Could you check a few things on this model? Use its own coordinates, in mm. Face numbers are marked on the shaded views. Round coordinates to 2 decimals unless told otherwise and drop trailing zeros. Write each loop counter-clockwise with the first axis right and the second up, starting at its lowest first coordinate (ties: lowest second). Pieces come first, ordered by that corner, then holes.
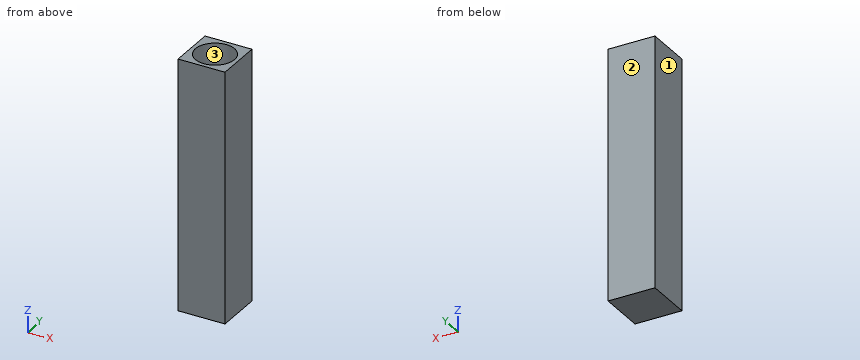
```python
from build123d import *

# Parameters (mm, degrees)
SKETCH1_W           = 76.2
SKETCH1_H           = 76.2
SKETCH1_R           = 31.75
BOSS_EXTRUDE1_DEPTH = 406.4
CUT_EXTRUDE1_START  = 406.4
SKETCH1_3_R         = 31.75
CUT_EXTRUDE1_DEPTH  = 304.8


with BuildPart() as part:
    # Sketch1 → Boss-Extrude1 (new body)
    with BuildSketch(Plane.XY):
        Rectangle(SKETCH1_W, SKETCH1_H)
        Circle(SKETCH1_R, mode=Mode.SUBTRACT)
        Circle(SKETCH1_R)
    extrude(amount=BOSS_EXTRUDE1_DEPTH)

    # Sketch1<3> → Cut-Extrude1 (cut)
    with BuildSketch(Plane.XY.offset(CUT_EXTRUDE1_START)):
        Circle(SKETCH1_3_R)
    extrude(amount=-CUT_EXTRUDE1_DEPTH, mode=Mode.SUBTRACT)


solid = part.part
```
Q1. Imagine slicing it at A-A, the plane y = -5.5. Write out the boundary of the cut face in (x, z), then the cut area to 3 significant figures.
Q2. Imagine slicing it at B-B, the plane x = 0. Write out the boundary of the cut face in (y, z), then the cut area to 3 significant figures.
Q3. If I drill on L1, parallel to Y at x = 0.5, z = 133.5; L2, parallel to Z at x = 24, y = 15.5; L3, parallel to X at y = -25, z = 248, over which ranges is the centre line in solid material (lowest first)?
Q4. We'd pull the mould along X, two halves only. Please class the marked faces 1, 2 and 3: pulls with the +X half, pulls with the -X half, needs draft (parallel to the pull), parting line crosses it, or undercut.
Q5. I'm going to push flat-ended pins straight in: pin 1 Ø12 at (x, y) = (13.5, -29) entering from -Z; pin 2 Ø1.5 at (x, y) = (-18.5, -3) entering from +Z. Where does each tip first touch, or does it pass through?
Results found:
1. outline: (-38.1, 0) - (38.1, 0) - (38.1, 406.4) - (31.27, 406.4) - (31.27, 101.6) - (-31.27, 101.6) - (-31.27, 406.4) - (-38.1, 406.4) - close
1. area: 11,900 mm2
2. outline: (-38.1, 0) - (38.1, 0) - (38.1, 406.4) - (31.75, 406.4) - (31.75, 101.6) - (-31.75, 101.6) - (-31.75, 406.4) - (-38.1, 406.4) - close
2. area: 11,600 mm2
3. L1: y = -38.1 to -31.75, 31.75 to 38.1
3. L2: z = 0 to 101.6
3. L3: x = -38.1 to -19.57, 19.57 to 38.1
4. face 1: pulls with the -X half
4. face 2: needs draft
4. face 3: undercut
5. pin 1: stops at z = 0
5. pin 2: stops at z = 101.6
